Part model, mm, in its own coordinate system. A direction names the side the tool comes from. Coordinates: 2 decimals unless noted, no trailing zeros. Order: outer loops, then holes, each group sorted by start corner. A loop starts at its lowest first (then second) coordinate and runs counter-clockwise, first axis right, second up.
1) Cut at D-D (y = 18.5). List the corners of the cut face in (x, z), and give its area (3 significant figures).
2) Cut at A-A (y = -8). List the corners of the cut face in (x, z).
3) Mould opens along X. For faces 5 (the flat face through (-5.1, 47, 68)), 6 (the flat face through (-1, 1, 6)), 7 (the flat face through (-47, -5.1, 68)), 8 (the flat face through (52, 0, 29)) say: +X half, -X half, draft (parallel to the pull), parting line (faces both ways), or undercut.
4) Cut at C-C (z = 12). List the corners of the cut face in (x, y).
5) Tool access for faces 1 (the flat face through (0, 47, 65)), 2 (the cylindrical face through (48.445, 12.773, 26.455)), 3 (the flat face through (-47, 5.1, 68)), 4 (the cylindrical face through (-47.289, -0.729, 27.152)): list every direction of +Z, -Z, +X, -X, +Y, -Y with a clear straight run to the whole face (end or side of a thin tool).
6) Pin check, flat tips, straight feed: pin 1 Ø4 at (y, z) = (-20.5, 55) entering from +X; pin 2 Ø5 at (x, y) = (3, 30) entering from +Z; pin 3 Ø1.6 at (x, y) = (-46.5, -2) entering from +Z. Stop position of each tip, or through.
7) Wall check: L1, parallel to X at y = 0, z = 30; L2, parallel to X at y = 0, z = 39; L3, parallel to Z at x = -48.55, y = 0. Give the ranges that are in metal, low to high.
8) Cut at B-B (x = 0). List the corners of the cut face in (y, z), and give its area (3 significant figures).
```python
from build123d import *

# Parameters (mm, degrees)
F0_R      = 50
F1_DEPTH  = 71
F2_R      = 45
F3_DEPTH  = 65
F4_W      = 10.2
F4_H      = 6
F5_DEPTH  = 50
F6_W      = 10.2
F6_H      = 6
F7_DEPTH  = 50
F8_W      = 10.2
F8_H      = 6
F9_DEPTH  = 50
F10_W     = 10.2
F10_H     = 6
F11_DEPTH = 50
F12_R     = 5.6
F13_DEPTH = 55
F14_R     = 5.6
F15_DEPTH = 56
F17_DEPTH = 52
F18_DEPTH = 55
F19_R     = 45
F20_DEPTH = 50


with BuildPart() as f1:
    # F0 (on Top) → F1 (new body)
    with BuildSketch(Plane.XY):
        Circle(F0_R)
    extrude(amount=F1_DEPTH)

    # F2 (on face) → F3 (cut)
    with BuildSketch(Plane.XY.offset(71)):
        Circle(F2_R)
    extrude(amount=-F3_DEPTH, mode=Mode.SUBTRACT)

    # F4 (on Front) → F5 (cut)
    with BuildSketch(Plane.XZ):
        with Locations((0, 68)):
            Rectangle(F4_W, F4_H)
    extrude(amount=-F5_DEPTH, mode=Mode.SUBTRACT)

    # F6 (on Front) → F7 (cut)
    with BuildSketch(Plane.XZ):
        with Locations((0, 68)):
            Rectangle(F6_W, F6_H)
    extrude(amount=F7_DEPTH, mode=Mode.SUBTRACT)

    # F8 (on Right) → F9 (cut)
    with BuildSketch(Plane.YZ):
        with Locations((0, 68)):
            Rectangle(F8_W, F8_H)
    extrude(amount=-F9_DEPTH, mode=Mode.SUBTRACT)

    # F10 (on Right) → F11 (cut)
    with BuildSketch(Plane.YZ):
        with Locations((0, 68)):
            Rectangle(F10_W, F10_H)
    extrude(amount=F11_DEPTH, mode=Mode.SUBTRACT)

    # F12 (on Right) → F13 (cut)
    with BuildSketch(Plane.YZ):
        with Locations((0, 21.6)):
            Circle(F12_R)
    extrude(amount=-F13_DEPTH, mode=Mode.SUBTRACT)

    # F14 (on Right) → F15 (cut)
    with BuildSketch(Plane.YZ):
        with Locations((-7.6, 28.6)):
            Circle(F14_R)
        with Locations((7.6, 28.6)):
            Circle(F14_R)
    extrude(amount=F15_DEPTH, mode=Mode.SUBTRACT)

    # F16 (on Right) → F17 (join)
    with BuildSketch(Plane.YZ):
        with BuildLine():
            ThreePointArc((0, 24.8768943744), (0.7464278423, 26.8786796564), (1, 29))
            ThreePointArc((1, 29), (0.7464278423, 31.1213203436), (0, 33.1231056256))
            ThreePointArc((0, 33.1231056256), (-1, 29), (0, 24.8768943744))
        make_face()
        with BuildLine():
            ThreePointArc((0, 33.1231056256), (0.7464278423, 31.1213203436), (1, 29))
            ThreePointArc((1, 29), (0.7464278423, 26.8786796564), (0, 24.8768943744))
            ThreePointArc((0, 24.8768943744), (10.1213203436, 20.2535721577), (17, 29))
            ThreePointArc((17, 29), (10.1213203436, 37.7464278423), (0, 33.1231056256))
        make_face()
        with BuildLine():
            ThreePointArc((0, 24.8768943744), (-1, 29), (0, 33.1231056256))
            ThreePointArc((0, 33.1231056256), (-17, 29), (0, 24.8768943744))
        make_face()
    extrude(amount=F17_DEPTH)

    # F14 (on Right) → F18 (cut)
    with BuildSketch(Plane.YZ):
        with Locations((-7.6, 28.6)):
            Circle(F14_R)
        with Locations((7.6, 28.6)):
            Circle(F14_R)
    extrude(amount=F18_DEPTH, mode=Mode.SUBTRACT)

    # F19 (on face) → F20 (cut)
    with BuildSketch(Plane.XY.offset(6)):
        Circle(F19_R)
    extrude(amount=F20_DEPTH, mode=Mode.SUBTRACT)


solid = f1.part
```
Geometry check:
1. outline: (-46.45, 0) - (46.45, 0) - (46.45, 71) - (41.02, 71) - (41.02, 6) - (-41.02, 6) - (-41.02, 71) - (-46.45, 71) - close
1. area: 1,260 mm2
2. outline: (-49.36, 0) - (49.36, 0) - (49.36, 20) - (52, 20) - (52, 23.01) - (44.28, 23.01) - (44.28, 6) - (-44.28, 6) - (-44.28, 71) - (-49.36, 71) - close; (44.28, 34.19) - (52, 34.19) - (52, 38) - (49.36, 38) - (49.36, 71) - (44.28, 71) - close
3. face 5: undercut
3. face 6: undercut
3. face 7: draft
3. face 8: +X half
4. outline: circle Ø100 at (0, 0); hole circle Ø90 at (0, 0)
5. face 1: +Z, +Y, -Y
5. face 2: +X
5. face 3: +Z, +X, -X
5. face 4: -X
6. pin 1: stops at x = 46.45
6. pin 2: stops at z = 6
6. pin 3: stops at z = 65
7. L1: x = -50 to -45, 45 to 52
7. L2: x = -50 to -45, 45 to 50
7. L3: z = 0 to 16, 27.2 to 65
8. outline: (-50, 0) - (50, 0) - (50, 65) - (45, 65) - (45, 6) - (-45, 6) - (-45, 65) - (-50, 65) - close
8. area: 1,190 mm2
